The listing builds one solid part. Answer for the finished solid, in the listing's coordinates (mm). A direction names the side the tool comes from. Round coordinates to 2 decimals unless told otherwise and drop trailing zeros. One line per item, written item: value. Start each with the question number.
1. For a pull along X with two mould halves and no side action, classify faces 4 (the cylindrical face through (-36.86, 0.22, 9.64)), 5 (the cylindrical face through (-18.326, 24.636, -35.635)), 6 (the flat face through (7, 25.4, -1)), 7 (the flat face through (4.762, 0, 0)) as released by +X, released by -X, zero draft, split by the parting line, or undercut.
2. A tool of negligible diameter and unlimited length cuts with its end or side. For faces 1 (the cylindrical face through (18.286, -24.676, -35.635)), 2 (the flat face through (-2.41, 0.36, 4.11)), 3 (the cylindrical face through (-18.286, -24.676, -35.635)), from which of +Z, -Z, +X, -X, +Y, -Y can it reach the whole face along a straight path? Write none if from no direction.
3. Flat-ended cylindrical pins translate along their axes: P1, Ø1.2, axis at y = 4, z = -35, coming from the -X side; P2, Ø8, axis at y = -6.5, z = -3, coming from the -X side; P3, Ø1.6, axis at y = 1.5, z = -1, coming from the -X side. Find the tip coordinate at first contact, or state that the pin passes through.
4. Straight lines are drawn through the part: line 1 (Y direction, x = 47, z = -2.5); line 2 (Y direction, x = -45, z = 13); line 3 (Z direction, x = 45, y = -6.5). For each, find the intervals that lie inside material, in ascending order.
from build123d import *

# Parameters (mm, degrees)
SKETCH1_R           = 38.1
SKETCH1_W           = 38.1
SKETCH1_H           = 6.35
BOSS_EXTRUDE1_DEPTH = 25.4
BOSS_EXTRUDE2_START = -25.4
SKETCH3_R           = 22.225
SKETCH3_R_2         = 15.875
BOSS_EXTRUDE2_DEPTH = 33.655
FILLET1_R           = 2.54


with BuildPart() as part:
    # Sketch1 → Boss-Extrude1 (new, symmetric)
    # profile 1 of 2: a face of its own
    with BuildSketch(Plane(origin=(0, 0, 0), x_dir=(1, 0, 0), z_dir=(0, 1, 0))):
        Circle(SKETCH1_R)
        Polygon((0, -5.499261314), (4.7625, -2.749630657), (4.7625, 2.749630657), (0, 5.499261314), (-4.7625, 2.749630657), (-4.7625, -2.749630657), align=None, mode=Mode.SUBTRACT)
    # profile 2 of 2: a face of its own
    with BuildSketch(Plane(origin=(0, 0, 0), x_dir=(1, 0, 0), z_dir=(0, 1, 0))):
        with Locations((0, 36.170567884)):
            Rectangle(SKETCH1_W, SKETCH1_H)
    extrude(amount=BOSS_EXTRUDE1_DEPTH, both=True)

    # Sketch3 → Boss-Extrude2 (add)
    with BuildSketch(Plane(origin=(36.801773982, 0, 9.861005618), x_dir=(-0.2588190451025214, 0, 0.9659258262890681), z_dir=(-0.9659258262890681, 0, -0.2588190451025214)).offset(BOSS_EXTRUDE2_START)):
        with Locations(Location((0, 0, 0), (0, 0, 180))):
            Circle(SKETCH3_R)
        with Locations(Location((0, 0, 0), (0, 0, 180))):
            Circle(SKETCH3_R_2, mode=Mode.SUBTRACT)
    boss_extrude2 = extrude(amount=BOSS_EXTRUDE2_DEPTH)

    # Mirror1: Boss-Extrude2 across plane
    add(boss_extrude2.mirror(Plane(origin=(0, 0, 0), x_dir=(0, 0, 1), z_dir=(1, 0, 0))))

    # Fillet1
    fillet1_edges = [part.edges().sort_by_distance(p)[0] for p in [
        (19.05, 25.4, -36.170567884),
        (0, -25.4, -39.345567884),
        (19.05, -25.4, -36.170567884),
        (0, -25.4, 38.1),
        (-19.05, -25.4, -36.170567884),
        (0, 25.4, -39.345567884),
        (-19.05, 0, -39.345567884),
        (19.05, 0, -39.345567884),
        (19.05, 0, -32.995567884),
        (-19.05, 0, -32.995567884),
        (-19.05, 25.4, -36.170567884),
        (0, 25.4, 38.1),
    ]]
    fillet(fillet1_edges, radius=FILLET1_R)


solid = part.part
Answer list:
1. face 4: undercut
1. face 5: released by -X
1. face 6: zero draft
1. face 7: undercut
2. face 1: -Z, +X, -Y
2. face 2: +Y, -Y
2. face 3: -Z, -X, -Y
3. P1: stops at x = -19.05
3. P2: stops at x = -67.04
3. P3: stops at x = -66.22
4. line 1: y = -16.77 to -6.28, 6.28 to 16.77
4. line 2: y = -22.21 to -15.85, 15.85 to 22.21
4. line 3: z = -9.95 to -2.94, 27.05 to 34.06
